from build123d import *

# Parameters (mm, degrees)
SKETCH1_R                = 12.5
SKETCH1_R_2              = 1.05
SKETCH1_R_3              = 5
BOSS_EXTRUDE1_DEPTH      = 2
BOSS_EXTRUDE5_START      = -2
BOSS_EXTRUDE5_DEPTH      = 2
BOSS_EXTRUDE6_DEPTH      = 50
BOSS_EXTRUDE6_DEPTH_BACK = 2
SKETCH9_W                = 25.04914064
SKETCH9_H                = 2
BOSS_EXTRUDE7_DEPTH      = 2
SKETCH13_R               = 2.5
CUT_EXTRUDE1_DEPTH       = 7
SKETCH15_W               = 1
SKETCH15_H               = 6
BOSS_EXTRUDE8_DEPTH      = 10
CUT_EXTRUDE2_START       = -1
CUT_EXTRUDE2_DEPTH       = 25
CUT_EXTRUDE3_DEPTH       = 5


# Read off the part's stored shape, not the designer's step: Cut-Extrude2
with BuildPart() as part:
    # Sketch1 → Boss-Extrude1 (new body)
    with BuildSketch(Plane.XY):
        Circle(SKETCH1_R)
        with Locations((-9.05, 0)):
            Circle(SKETCH1_R_2, mode=Mode.SUBTRACT)
        with Locations((9.05, 0)):
            Circle(SKETCH1_R_2, mode=Mode.SUBTRACT)
        Circle(SKETCH1_R_3, mode=Mode.SUBTRACT)
    extrude(amount=BOSS_EXTRUDE1_DEPTH)

    # Sketch2 → Boss-Extrude5 (add)
    with BuildSketch(Plane.XY.offset(2).offset(BOSS_EXTRUDE5_START)):
        with BuildLine():
            ThreePointArc((12.5, 0), (8.838834759, -8.838834771), (-1.6e-08, -12.5))
            Line((-1.6e-08, -12.5), (12.5, -12.5))
            Line((12.5, -12.5), (12.5, 0))
        make_face()
        with BuildLine():
            ThreePointArc((-1.6e-08, -12.5), (-8.838834771, -8.838834759), (-12.5, 0))
            Line((-12.5, 0), (-12.5, -12.5))
            Line((-12.5, -12.5), (-1.6e-08, -12.5))
        make_face()
    extrude(amount=BOSS_EXTRUDE5_DEPTH)

    # Sketch9 → Boss-Extrude6 (add, two sides: drawn at the far end of the back side and taken through both)
    with BuildSketch(Plane(origin=(0, 0, 0), x_dir=(-1, 0, 0), z_dir=(0, 0, -1)).offset(-BOSS_EXTRUDE6_DEPTH_BACK)):
        with Locations((0.02457032, -13.5)):
            Rectangle(SKETCH9_W, SKETCH9_H)
    extrude(amount=BOSS_EXTRUDE6_DEPTH + BOSS_EXTRUDE6_DEPTH_BACK)

    # Sketch12 → Boss-Extrude7 (add)
    with BuildSketch(Plane(origin=(0, -12.5, 0), x_dir=(1, 0, 0), z_dir=(0, 1, 0))):
        Polygon((-12.54914064, 50), (-32.54914064, 50), (-32.54914064, 10), (-12.5, -2), (-12.54914064, 0), align=None)
        Polygon((12.5, 50), (32.5, 50), (32.5, 10), (12.5, -2), (12.5, 0), align=None)
    extrude(amount=-BOSS_EXTRUDE7_DEPTH)

    # Sketch13 → Cut-Extrude1 (cut)
    with BuildSketch(Plane(origin=(0, -12.5, 0), x_dir=(1, 0, 0), z_dir=(0, 1, 0))):
        with Locations(Location((-25, 20, 0), (0, 0, 270))):
            Circle(SKETCH13_R)
        with Locations(Location((-25, 40, 0), (0, 0, 270))):
            Circle(SKETCH13_R)
        with Locations(Location((25, 40, 0), (0, 0, 90))):
            Circle(SKETCH13_R)
        with Locations(Location((25, 20, 0), (0, 0, 90))):
            Circle(SKETCH13_R)
    extrude(amount=-CUT_EXTRUDE1_DEPTH, mode=Mode.SUBTRACT)

    # Sketch15 → Boss-Extrude8 (add)
    with BuildSketch(Plane(origin=(0, 0, 0), x_dir=(-1, 0, 0), z_dir=(0, 0, -1))):
        with Locations((12, -9.5)):
            Rectangle(SKETCH15_W, SKETCH15_H)
        with Locations((-12, -9.5)):
            Rectangle(SKETCH15_W, SKETCH15_H)
    extrude(amount=BOSS_EXTRUDE8_DEPTH)

    # Cut-Extrude2 outline → Cut-Extrude2 (cut)
    with BuildSketch(Plane(origin=(-11.5, 0, 0), x_dir=(0, 0, -1), z_dir=(1, 0, 0)).offset(CUT_EXTRUDE2_START)):
        Polygon((10, -6.5), (0, -6.5), (10, -12.5), align=None)
    extrude(amount=CUT_EXTRUDE2_DEPTH, mode=Mode.SUBTRACT)

    # Sketch17 → Cut-Extrude3 (cut)
    with BuildSketch(Plane(origin=(0, -12.5, 0), x_dir=(1, 0, 0), z_dir=(0, 1, 0))):
        with BuildLine():
            Line((7.47542968, 40), (-7.52457032, 40))
            ThreePointArc((-7.52457032, 40), (-11.060104226, 38.535533906), (-12.52457032, 35))
            Line((-12.52457032, 35), (-12.52457032, 25))
            ThreePointArc((-12.52457032, 25), (-11.060104226, 21.464466094), (-7.52457032, 20))
            Line((-7.52457032, 20), (7.47542968, 20))
            ThreePointArc((7.47542968, 20), (11.010963586, 21.464466094), (12.47542968, 25))
            Line((12.47542968, 25), (12.47542968, 35))
            ThreePointArc((12.47542968, 35), (11.010963586, 38.535533906), (7.47542968, 40))
        make_face()
    extrude(amount=-CUT_EXTRUDE3_DEPTH, mode=Mode.SUBTRACT)


solid = part.part
Part model, mm, in its own coordinate system. A direction names the side the tool comes from. Coordinates: 2 decimals unless noted, no trailing zeros. Order: outer loops, then holes, each group sorted by start corner. A loop starts at its lowest first (then second) coordinate and runs counter-clockwise, first axis right, second up. Notation, with made-up numbers: M -1,37.5 L 18,37.5 A27 cw 18,60.5 Z; hole C 45,-25 d2. An arc over 180 degrees is marked long. Use a Markdown table: item, result.
(1) Cut at B-B on y = 2. Write the cut outline in (x, z), then the cut area to 3 significant figures.
A:
| item | result |
|---|---|
| outline | M -12.34,0 L -4.58,0 L -4.58,2 L -12.34,2 Z; M 4.58,0 L 12.34,0 L 12.34,2 L 4.58,2 Z |
| area | 31.0 mm^2 |
(2) Cut at A-A on x = 0. Write the cut outline in (y, z).
A:
| item | result |
|---|---|
| outline | M -14.5,-50 L -12.5,-50 L -12.5,-40 L -14.5,-40 Z; M -14.5,-20 L -12.5,-20 L -12.5,0 L -5,0 L -5,2 L -14.5,2 Z; M 5,0 L 12.5,0 L 12.5,2 L 5,2 Z |
(3) Cut at D-D on x = -25. Write the cut outline in (y, z).
A:
| item | result |
|---|---|
| outline | M -14.5,-50 L -12.5,-50 L -12.5,-42.5 L -14.5,-42.5 Z; M -14.5,-37.5 L -12.5,-37.5 L -12.5,-22.5 L -14.5,-22.5 Z; M -14.5,-17.5 L -12.5,-17.5 L -12.5,-5.48 L -14.5,-5.48 Z |
(4) Tool access for faces 1 (the flat face through (11.5, -10, -4)), 2 (the flat face through (-12.5, -8, -1)), 3 (the flat face through (0, -7, 2)), 4 (the cylindrical face through (11.05, -13.486, -38.496)), 5 (the cylindrical face through (-1.08, -4.88, 0.99)): list every direction of +Z, -Z, +X, -X, +Y, -Y with a clear straight run to the whole face (end or side of a thin tool).
A:
| item | result |
|---|---|
| face 1 | -Z, +Y |
| face 2 | +Z, -Z, -X, +Y |
| face 3 | +Z, +X, -X, +Y, -Y |
| face 4 | +Y, -Y |
| face 5 | +Z, -Z |
(5) Probe L1, parallel to Y at x = -11.5, z = -14; L2, parallel to Z at x = -8, y = 0.75. List the from-to ranges inside material, lowest first.
A:
| item | result |
|---|---|
| L1 | y = -14.5 to -12.5 |
| L2 | z = 0 to 2 |
(6) Flat gauge pins, fed straight in: pin 1 (4 mm diameter, centred on x = -25, z = -20, fed in from +Y) (3 decimals); pin 2 (5 mm diameter, centred on y = -9.5, z = -7.5, fed in from -X); pin 3 (8 mm diameter, centred on x = 19.5, z = -36, fed in from +Y); pin 4 (2.5 mm diameter, centred on x = -9.05, y = 0, fed in from -Z). Where does each tip first touch, or does it go through?
A:
| item | result |
|---|---|
| pin 1 | passes through |
| pin 2 | stops at x = -12.5 |
| pin 3 | stops at y = -12.5 |
| pin 4 | stops at z = 0 |
(7) Pull direction Y, two halves, no side cores. Call faces 6 (the flat face through (0, -13, -40)), 7 (the flat face through (0, -14.5, -19)), 8 (the cylindrical face through (-8, 0, 1)): released by +Y, released by -Y, zero draft, split by the parting line, or undercut.
A:
| item | result |
|---|---|
| face 6 | zero draft |
| face 7 | released by -Y |
| face 8 | undercut |
(8) Cut at C-C on z = -9. Write the cut outline in (x, y).
A:
| item | result |
|---|---|
| outline | M -30.88,-14.5 L 30.83,-14.5 L 30.83,-12.5 L 12.5,-12.5 L 12.5,-11.9 L 11.5,-11.9 L 11.5,-12.5 L -11.5,-12.5 L -11.5,-11.9 L -12.5,-11.9 L -12.5,-12.5 L -30.88,-12.5 Z |
